Check sheet for the modelled part. Datum: model origin and axes. Units: mm. Face numbers are marked on the shaded views. Round coordinates to 2 decimals unless told otherwise and drop trailing zeros. Write each loop counter-clockwise with the first axis right and the second up, starting at its lowest first coordinate (ties: lowest second). Pieces come first, ordered by that corner, then holes. Notation, with made-up numbers: M 27.5,4 L 78.5,4 A20 cw 78.5,26 Z; hole C -22.75,75 d5. An arc over 180 degrees is marked long. One line per item, written item: value.
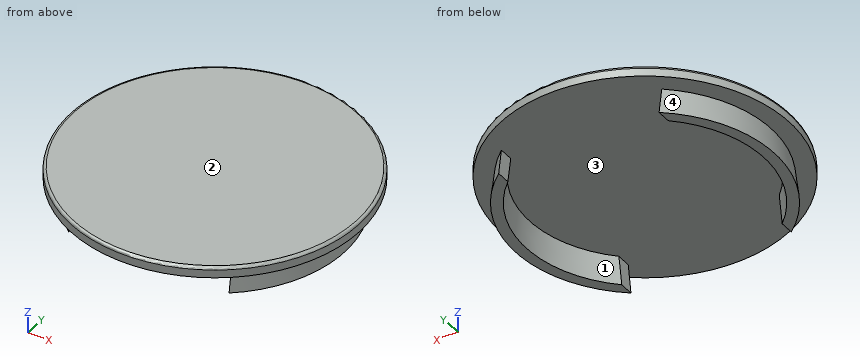
from build123d import *

# Parameters (mm, degrees)
F0_R          = 27
F0_R_2        = 23.65
F1_DEPTH      = 2
F2_DEPTH      = 5
F2_TAPER      = -7
F3_T          = -2
F4_W          = 15
F4_H          = 7.3000405619
F5_DEPTH      = 25
F5_DEPTH_BACK = 25
F6_R          = 0.5


with BuildPart() as f1:
    # F0 (on Top) → F1 (new body)
    with BuildSketch(Plane.XY):
        Circle(F0_R)
        Circle(F0_R_2, mode=Mode.SUBTRACT)
        Circle(F0_R_2)
    extrude(amount=F1_DEPTH)

    # F0 (on Top) → F2 (join)
    with BuildSketch(Plane.XY):
        Circle(F0_R_2)
    extrude(amount=-F2_DEPTH, taper=F2_TAPER)

    # F3
    f3_openings = [f1.faces().sort_by_distance(p)[0] for p in [
        (0, 0, -5),
    ]]
    offset(amount=F3_T, openings=f3_openings, kind=Kind.INTERSECTION)

    # F4 (on Front) → F5 (cut, two sides)
    with BuildSketch(Plane.XZ) as f5_sk:
        with Locations((7.5, -3.6500202809)):
            Rectangle(F4_W, F4_H)
        with Locations((-7.5, -3.6500202809)):
            Rectangle(F4_W, F4_H)
    extrude(amount=-F5_DEPTH, mode=Mode.SUBTRACT)
    extrude(f5_sk.sketch, amount=F5_DEPTH_BACK, mode=Mode.SUBTRACT)

    # F6
    f6_edges = [f1.edges().sort_by_distance(p)[0] for p in [
        (-27, 0, 2),
    ]]
    fillet(f6_edges, radius=F6_R)


solid = f1.part
Q1. Scan lines: line 1 (Z direction, x = 5, y = -23); line 2 (Y direction, x = 17.5, z = -2.5); line 3 (X direction, y = 9.5, z = -3.25). Record each from-to range of solid material in increasing order. Write a range as [from, to].
Completed:
line 1: [0, 2]
line 2: [-16.36, -13.24], [13.24, 16.36]
line 3: [-22.09, -19.88], [19.88, 22.09]
Q2. Sectioned sample at A-A on z = -1. Enter the section's corners in (x, y).
Completed:
outline: M -15,-18.44 L -15,-15.76 A21.76 cw -15,15.76 L -15,18.44 A23.77 ccw Z; M 15,-18.44 A23.77 ccw 15,18.44 L 15,15.76 A21.76 cw 15,-15.76 Z
Q3. Sectioned sample at B-B on x = 0. Enter the section's corners in (y, z), and give its area (3 significant figures).
Completed:
outline: M -27,0 L 27,0 L 27,1.5 A0.5 ccw 26.5,2 L -26.5,2 A0.5 ccw -27,1.5 Z
area: 108 mm^2
Q4. Sectioned sample at C-C on y = 0. Enter the section's corners in (x, z), and give its area (3 significant figures).
Completed:
outline: M -27,0 L -23.65,0 L -24.26,-5 L -22.25,-5 L -21.63,0 L 21.63,0 L 22.25,-5 L 24.26,-5 L 23.65,0 L 27,0 L 27,1.5 A0.5 ccw 26.5,2 L -26.5,2 A0.5 ccw -27,1.5 Z
area: 128 mm^2
Q5. Depth check by flat-ended pin: P1, Ø3, axis at y = 17.5, z = -2.5, coming from the -X side; P2, Ø1, axis at y = -17, z = -2.5, coming from the -X side; P3, Ø1.7, axis at y = 17.5, z = -3.5, coming from the +X side. Enter the tip coordinate at first touch or a pass-through.
Completed:
P1: x = -17.85
P2: x = -17.38
P3: x = 17.41
Q6. Draft check along Y on the marked faces 1, 2, 3 and 4. Enter one of: pulls with the +Y half, pulls with the -Y half, needs draft (parallel to the pull), parting line crosses it, or undercut.
Completed:
face 1: undercut
face 2: needs draft
face 3: undercut
face 4: parting line crosses it
